Design review of the part built by this model. Coordinates are the model's own, in mm. A direction names the side the tool comes from. Coordinates: 2 decimals unless noted, no trailing zeros. Write each loop counter-clockwise with the first axis right and the second up, starting at its lowest first coordinate (ties: lowest second). Pieces come first, ordered by that corner, then holes. Notation, with made-up numbers: M -4,5.5 L 20,5.5 A15 cw 20,23.5 Z; hole C -36,29 d5. An arc over 180 degrees is marked long. Write item = value, one per line.
```python
from build123d import *

# Parameters (mm, degrees)
SKETCH1_W           = 34.4
SKETCH1_H           = 12.2
BOSS_EXTRUDE1_DEPTH = 1.6
SKETCH8_R           = 1.6
CUT_EXTRUDE3_DEPTH  = 24.175783188
FILLET2_R           = 3
FILLET3_R           = 6.1
SKETCH2_W           = 8.6
SKETCH2_H           = 6
BOSS_EXTRUDE2_DEPTH = 3.5
SKETCH3_R           = 0.7
CUT_EXTRUDE1_DEPTH  = 6
BOSS_EXTRUDE3_DEPTH = 3.4
SKETCH5_W           = 6.1
SKETCH5_H           = 1.6
BOSS_EXTRUDE4_DEPTH = 9.2
BOSS_EXTRUDE5_DEPTH = 1.6
SKETCH7_R           = 1.6
CUT_EXTRUDE2_DEPTH  = 1.6
FILLET1_R           = 20


# Some blends are built 0.0001 mm under size
with BuildPart() as part:
    # Sketch1 → Boss-Extrude1 (new body)
    with BuildSketch(Plane(origin=(0, 0, 0), x_dir=(1, 0, 0), z_dir=(0, 1, 0))):
        with Locations((3.513069909, 4.172568389)):
            Rectangle(SKETCH1_W, SKETCH1_H)
    extrude(amount=BOSS_EXTRUDE1_DEPTH)

    # Sketch8 → Cut-Extrude3 (cut, through all)
    with BuildSketch(Plane(origin=(0, 1.6, 0), x_dir=(1, 0, 0), z_dir=(0, 1, 0))):
        with Locations(Location((14.613069909, 4.172568389, 0), (0, 0, 270))):
            Circle(SKETCH8_R)
        with BuildLine():
            Line((5.763069909, 10.272568389), (-2.336930091, 10.272568389))
            ThreePointArc((-2.336930091, 10.272568389), (1.713069909, 6.222568389), (5.763069909, 10.272568389))
        make_face()
    extrude(amount=-CUT_EXTRUDE3_DEPTH, mode=Mode.SUBTRACT)

    # Fillet2
    fillet2_edges = [part.edges().sort_by_distance(p)[0] for p in [
        (-13.686930091, 0.8, -10.272568389),
    ]]
    fillet(fillet2_edges, radius=FILLET2_R)

    # Fillet3
    fillet3_edges = [part.edges().sort_by_distance(p)[0] for p in [
        (20.713069909, 0.8, 1.927431611),
        (20.713069909, 0.8, -10.272568389),
    ]]
    fillet(fillet3_edges, radius=FILLET3_R - 0.0001)  # a hair under: the kernel refuses the full size

    # Sketch2 → Boss-Extrude2 (add)
    with BuildSketch(Plane(origin=(0, 1.6, 0), x_dir=(1, 0, 0), z_dir=(0, 1, 0))):
        with Locations((-9.386930091, 1.072568389)):
            Rectangle(SKETCH2_W, SKETCH2_H)
    extrude(amount=BOSS_EXTRUDE2_DEPTH)

    # Sketch3 → Cut-Extrude1 (cut)
    with BuildSketch(Plane.XY.offset(1.927431611)):
        with Locations((-11.986930091, 3.35)):
            Circle(SKETCH3_R)
        with Locations((-6.786930091, 3.35)):
            Circle(SKETCH3_R)
        with Locations((-9.386930091, 3.35)):
            Circle(SKETCH3_R)
    extrude(amount=-CUT_EXTRUDE1_DEPTH, mode=Mode.SUBTRACT)



with BuildPart() as body_2:
    # Sketch4 → Boss-Extrude3 (new body)
    with BuildSketch(Plane.XZ):
        with BuildLine():
            Line((-13.686930091, 1.927431611), (-13.686930091, -4.172568389))
            Line((-13.686930091, -4.172568389), (-19.786930091, -4.172568389))
            ThreePointArc((-19.786930091, -4.172568389), (-18.000281456, 0.140782976), (-13.686930091, 1.927431611))
        make_face()
    extrude(amount=-BOSS_EXTRUDE3_DEPTH)


with BuildPart() as part_1:
    add(part.part)

    add(body_2.part)  # Boss-Extrude4 merges body 2
    # Sketch5 → Boss-Extrude4 (add)
    with BuildSketch(Plane(origin=(0, 0, -4.172568389), x_dir=(-1, 0, 0), z_dir=(0, 0, -1))):
        with Locations((16.736930091, 2.6)):
            Rectangle(SKETCH5_W, SKETCH5_H)
    extrude(amount=BOSS_EXTRUDE4_DEPTH)

    # Sketch6 → Boss-Extrude5 (add)
    with BuildSketch(Plane(origin=(0, 3.4, 0), x_dir=(1, 0, 0), z_dir=(0, 1, 0))):
        with BuildLine():
            Line((-19.786930091, 13.372568389), (-13.686930091, 13.372568389))
            ThreePointArc((-13.686930091, 13.372568389), (-16.736930091, 16.422568389), (-19.786930091, 13.372568389))
        make_face()
    extrude(amount=-BOSS_EXTRUDE5_DEPTH)

    # Sketch7 → Cut-Extrude2 (cut)
    with BuildSketch(Plane(origin=(0, 3.4, 0), x_dir=(1, 0, 0), z_dir=(0, 1, 0))):
        with Locations(Location((-16.686930091, 10.272568389, 0), (0, 0, 270))):
            Circle(SKETCH7_R)
    extrude(amount=-CUT_EXTRUDE2_DEPTH, mode=Mode.SUBTRACT)

    # Fillet1
    # the kernel refuses this fillet: 20 mm, written as the material it takes off along each edge
    with BuildSketch(Plane(origin=(5.763069909, 23.72525, -10.272568389), x_dir=(-0.47132268480502076, 0, 0.8819608419811998), z_dir=(0, -1, 0))) as fillet1_piece_1:
        with BuildLine():
            CenterArc((13.244167443, -17.63921684), FILLET1_R, 118.12018917, 32.428171428)
            Line((-4.171252893, -7.805441648), (-4.5195613, -7.608766144))
            ThreePointArc((-4.5195613, -7.608766144), (-2.438410783, -3.71419175), (-0.352784337, 0.188529074))
            Line((-0.352784337, 0.188529074), (0.188529074, 0.352784337))
            ThreePointArc((0.188529074, 0.352784337), (1.908856873, -0.07805859), (3.629184673, 0.352784337))
            Line((3.629184673, 0.352784337), (3.817713747, 0))
        make_face()
    extrude(amount=45.8505, mode=Mode.SUBTRACT)


solid = part_1.part
```
Q1. For P1, Ø1.7, axis at x = -11, y = 3, coming from the -Z side; P2, Ø0.5, axis at y = 2.5, z = -8.5, coming from the +X side; P3, Ø5, axis at x = 2, z = -0.5, coming from the +Y side; P4, Ø2, axis at y = 4.5, z = -12, coming from the -X side, all flat-tipped, find the tip position at first contact; note any pin that passes through.
Check result:
P1 = -4.07
P2 = -13.69
P3 = 1.6
P4 = through
Q2. Consider section A-A, the plane z = 0. State the section outline as (x, y) points, and give its area (3 significant figures).
Check result:
outline = M -18.14,0 L 19.06,0 L 19.06,1.6 L -5.09,1.6 L -5.09,5.1 L -13.69,5.1 L -13.69,3.4 L -18.14,3.4 Z; hole C -11.99,3.35 d1.4; hole C -9.39,3.35 d1.4; hole C -6.79,3.35 d1.4
area = 93.0 mm²
Q3. Machinability: for faces 1 (the flat face through (-13.687, 4, -1)), 2 (the flat face through (-17, 1, -4.173)), 3 (the flat face through (-5.087, 3, -1)), 4 (the cylindrical face through (8.973, 0.811, -9.323)), which of the approach directions +Z, -Z, +X, -X, +Y, -Y give a long, thin tool a straight path to every point of the face, cutting with its end or side? Answer none if there is none.
Check result:
face_1 = +Z, -Z, -X, +Y
face_2 = -Z, -X, -Y
face_3 = +Z, -Z, +X, +Y
face_4 = -Z, +Y, -Y
Q4. Consider section D-D, the plane z = -13.75. State the section outline as (x, y) points.
Check result:
outline = M -19.76,1.8 L -13.71,1.8 L -13.71,3.4 L -19.76,3.4 Z
Q5. The part is to be moulded in two halves that separate along Y. For faces 5 (the cylindrical face through (-6.46, 2.73, -1.03)), 6 (the flat face through (-9, 5.1, -1)), 7 (the flat face through (-18, 1.8, -9)), 8 (the cylindrical face through (-8.74, 3.08, -1.03)), say which applies: +Y half, -Y half, draft (parallel to the pull), parting line (faces both ways), or undercut.
Check result:
face_5 = undercut
face_6 = +Y half
face_7 = -Y half
face_8 = undercut
Q6. Wall thickness on line 1 (Y direction, x = 14.5, z = -0.75); line 2 (Y direction, x = -9.5, z = -1); line 3 (Y direction, x = -14, z = -5.25): over which ranges is each line inside the solid? List them lowest first.
Check result:
line_1 = 0 to 1.6
line_2 = 0 to 2.66, 4.04 to 5.1
line_3 = 1.8 to 3.4
Q7. Consider section C-C, the plane x = -5.5. State the section outline as (y, z) points.
Check result:
outline = M 0,-10.27 L 1.6,-10.27 L 1.6,-4.07 L 5.1,-4.07 L 5.1,1.93 L 0,1.93 Z
